```python
from build123d import *

# Parameters (mm, degrees)
SKETCH1_R           = 8.75
BOSS_EXTRUDE1_DEPTH = 3
BOSS_EXTRUDE2_DEPTH = 10
SCALE1_SCALE        = 1.9


with BuildPart() as part:
    # Sketch1 → Boss-Extrude1 (new body)
    with BuildSketch(Plane.XY):
        Circle(SKETCH1_R)
    extrude(amount=BOSS_EXTRUDE1_DEPTH)

    # Sketch2 → Boss-Extrude2 (add)
    with BuildSketch(Plane.XY.offset(3)):
        with BuildLine():
            ThreePointArc((4.829991895, 5.737697996), (3.826186326, 5.132311911), (2.976672459, 4.324571779))
            ThreePointArc((2.976672459, 4.324571779), (2.440108702, 4.648480345), (1.868768811, 4.906139331))
            ThreePointArc((1.868768811, 4.906139331), (2.051102492, 6.064099762), (1.979255999, 7.234123699))
            ThreePointArc((1.979255999, 7.234123699), (1.795356309, 7.281943128), (1.610304214, 7.325088418))
            ThreePointArc((1.610304214, 7.325088418), (1.002815466, 6.322553954), (0.62598385, 5.212546807))
            ThreePointArc((0.62598385, 5.212546807), (0.000352422, 5.249999988), (-0.625284028, 5.212630803))
            ThreePointArc((-0.625284028, 5.212630803), (-1.001966616, 6.322688531), (-1.609320762, 7.325304546))
            ThreePointArc((-1.609320762, 7.325304546), (-1.794378647, 7.2821841), (-1.978284756, 7.234389361))
            ThreePointArc((-1.978284756, 7.234389361), (-2.050288332, 6.06437508), (-1.868110115, 4.90639018))
            ThreePointArc((-1.868110115, 4.90639018), (-2.439484593, 4.648807903), (-2.976091832, 4.324971377))
            ThreePointArc((-2.976091832, 4.324971377), (-3.825497247, 5.132825554), (-4.82922153, 5.738346401))
            ThreePointArc((-4.82922153, 5.738346401), (-4.97304308, 5.614164455), (-5.113672529, 5.486378884))
            ThreePointArc((-5.113672529, 5.486378884), (-4.633695781, 4.41692096), (-3.934242565, 3.476238691))
            ThreePointArc((-3.934242565, 3.476238691), (-4.320465088, 2.982629951), (-4.645112863, 2.44651313))
            ThreePointArc((-4.645112863, 2.44651313), (-5.772652562, 2.7670941), (-6.942805845, 2.83680225))
            ThreePointArc((-6.942805845, 2.83680225), (-7.012443275, 2.66000739), (-7.077579552, 2.481505124))
            ThreePointArc((-7.077579552, 2.481505124), (-6.15557937, 1.757603477), (-5.099087457, 1.249722811))
            ThreePointArc((-5.099087457, 1.249722811), (-5.211679097, 0.633167423), (-5.249994516, 0.007588209))
            ThreePointArc((-5.249994516, 0.007588209), (-6.397362742, -0.232545265), (-7.46587701, -0.71461911))
            ThreePointArc((-7.46587701, -0.71461911), (-7.445377224, -0.90352531), (-7.420098394, -1.091851556))
            ThreePointArc((-7.420098394, -1.091851556), (-6.267293907, -1.304359781), (-5.095792863, -1.263089504))
            ThreePointArc((-5.095792863, -1.263089504), (-4.908960234, -1.861346132), (-4.652165695, -2.43307508))
            ThreePointArc((-4.652165695, -2.43307508), (-5.556514215, -3.178911313), (-6.278605726, -4.102329843))
            ThreePointArc((-6.278605726, -4.102329843), (-6.172664978, -4.260071251), (-6.062762116, -4.415078202))
            ThreePointArc((-6.062762116, -4.415078202), (-4.94324694, -4.067509932), (-3.925113535, -3.486543236))
            ThreePointArc((-3.925113535, -3.486543236), (-3.48165774, -3.92944772), (-2.988581778, -4.316350189))
            ThreePointArc((-2.988581778, -4.316350189), (-3.442735244, -5.397027088), (-3.652981535, -6.550246247))
            ThreePointArc((-3.652981535, -6.550246247), (-3.485869574, -6.640686208), (-3.316520101, -6.726863639))
            ThreePointArc((-3.316520101, -6.726863639), (-2.486761671, -5.898842577), (-1.855237999, -4.91127193))
            ThreePointArc((-1.855237999, -4.91127193), (-1.256749416, -5.09736019), (-0.640349792, -5.210801488))
            ThreePointArc((-0.640349792, -5.210801488), (-0.540267119, -6.378748999), (-0.190503298, -7.497580176))
            ThreePointArc((-0.190503298, -7.497580176), (-0.00050346, -7.499999983), (0.189496701, -7.497605685))
            ThreePointArc((0.189496701, -7.497605685), (0.539410728, -6.378821476), (0.639650205, -5.210887412))
            ThreePointArc((0.639650205, -5.210887412), (1.256065053, -5.09752887), (1.854578614, -4.911520962))
            ThreePointArc((1.854578614, -4.911520962), (2.485969693, -5.899176387), (3.315616949, -6.727308842))
            ThreePointArc((3.315616949, -6.727308842), (3.48497799, -6.641154147), (3.652102092, -6.550736623))
            ThreePointArc((3.652102092, -6.550736623), (3.44201063, -5.397489248), (2.988002255, -4.316751385))
            ThreePointArc((2.988002255, -4.316751385), (3.481130156, -3.929915118), (3.92464541, -3.487070175))
            ThreePointArc((3.92464541, -3.487070175), (4.942700807, -4.068173557), (6.06216931, -4.415892125))
            ThreePointArc((6.06216931, -4.415892125), (6.172092982, -4.260899931), (6.278054907, -4.103172747))
            ThreePointArc((6.278054907, -4.103172747), (5.556087377, -3.17965728), (4.651838998, -2.433699639))
            ThreePointArc((4.651838998, -2.433699639), (4.908710292, -1.862005173), (5.09562324, -1.263773634))
            ThreePointArc((5.09562324, -1.263773634), (6.267118732, -1.305201192), (7.41995174, -1.092847739))
            ThreePointArc((7.41995174, -1.092847739), (7.445255854, -0.904524889), (7.465781001, -0.715621443))
            ThreePointArc((7.465781001, -0.715621443), (6.397331464, -0.233404148), (5.249995488, 0.006883365))
            ThreePointArc((5.249995488, 0.006883365), (5.211764057, 0.632467717), (5.099255194, 1.249038216))
            ThreePointArc((5.099255194, 1.249038216), (6.155815283, 1.756777037), (7.077912646, 2.480554893))
            ThreePointArc((7.077912646, 2.480554893), (7.012800334, 2.659065903), (6.94318664, 2.83587011))
            ThreePointArc((6.94318664, 2.83587011), (5.773024009, 2.766319061), (4.64544128, 2.445889473))
            ThreePointArc((4.64544128, 2.445889473), (4.320865485, 2.982049876), (3.934709236, 3.475710464))
            ThreePointArc((3.934709236, 3.475710464), (4.634288738, 4.416298818), (5.114409063, 5.485692293))
            ThreePointArc((5.114409063, 5.485692293), (4.973796771, 5.613496743), (4.829991895, 5.737697996))
        make_face()
    extrude(amount=BOSS_EXTRUDE2_DEPTH)


with BuildPart() as part_1:
    # Scale1: scaled about (0, 0, 5.507121535)
    add(part.part.scale(SCALE1_SCALE).moved(Location((0, 0, -4.956409381))))


solid = part_1.part
```
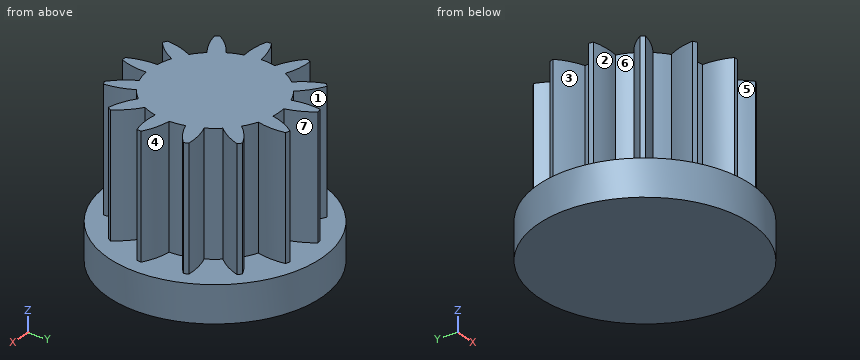
Source: CAD feature listing. Evaluate the final solid. Frame: model axes, mm. Face numbers are marked on the shaded views. A direction names the side the tool comes from. Give positions to 0.01 mm unless a question says otherwise; leave off trailing zeros. Write each loop counter-clockwise with the first axis right and the second up, starting at its lowest first coordinate (ties: lowest second). Pieces come first, ordered by that corner, then holes. Notation, with made-up numbers: (-11.5, 29.5) - (3.5, 29.5) arc R19 cw to (3.5, 51.5) - close; hole circle Ø3 at (-6.75, 88.25). An arc over 180 degrees is marked (long way). One line per item, written item: value. Start each with the question number.
Q1. Section query A-A, the plane x = 2. Return the cut outline in (y, z), then the cut area to 3 significant figures.
Q2. Draft query along Y for the marked faces 5, 6 and 7. Return one class per face: +Y half, -Y half, draft (parallel to the pull), parting line (faces both ways), or undercut.
Q3. Set-up query: the marked faces 1, 2, 3 and 4. Return all of +Z, -Z, +X, -X, +Y, -Y with unobstructed straight access to the full face (end or side cutting, diameter ignored); none if empty.
Q4. First-contact query: pin 1 Ø10 at (x, z) = (8.5, 0) entering from +Y; pin 2 Ø1.5 at (x, z) = (-5.5, 2) entering from +Y; pin 3 Ø6 at (y, z) = (4, 2) entering from -X. Flat tips, straight axial feed; report the tip coordinate or a pass-through.
Q5. Section query B-B, the plane z = -1.5. Return the cut outline in (x, y) (3 decimals), then the cut area to 3 significant figures.
Q6. Material intervals for probe 1 along X at (y, z) = (-10.5, 10.5); probe 2 along X at (y, z) = (-11.5, 12.25); probe 3 along Z at (x, y) = (-13, -0.5), sorted ascending. Write a range as from..to.
Answer:
1. outline: (-16.5, -4.96) - (16.5, -4.96) - (16.5, 0.74) - (12.21, 0.74) - (12.21, 19.74) - (-9.77, 19.74) - (-9.77, 0.74) - (-16.5, 0.74) - close
1. area: 606 mm2
2. face 5: -Y half
2. face 6: undercut
2. face 7: +Y half
3. face 1: +Z, +Y
3. face 2: +Z
3. face 3: +Z, -X
3. face 4: +Z, +X
4. pin 1: stops at y = 16.25
4. pin 2: stops at y = 8.86
4. pin 3: stops at x = -16.58
5. outline: circle Ø33.25 at (0, 0)
5. area: 868 mm2
6. probe 1: x = -6.61..-4.2, -1.21..1.21, 4.2..6.61
6. probe 2: x = -6.83..-4.97, -1.13..1.13, 4.97..6.83
6. probe 3: z = -4.96..0.74
